Check sheet for the modelled part. Datum: model origin and axes. Units: mm. Round coordinates to 2 decimals unless told otherwise and drop trailing zeros. Order: outer loops, then holes, each group sorted by start corner. A loop starts at its lowest first (then second) coordinate and runs counter-clockwise, first axis right, second up.
(1) Sectioned sample at B-B, the plane y = 107. Enter the section's corners in (x, z), and give its area (3 significant figures).
(2) Thickness scan on probe 1 along X at (y, z) = (259, 5.75); probe 2 along Z at (x, y) = (-16.5, 148). Record the ranges inside material, lowest first.
(3) Sectioned sample at A-A, the plane z = 4.75. Enter the section's corners in (x, y).
(4) Depth check by flat-ended pin: pin 1 (2.5 mm diameter, centred on y = 215, z = 6.5, fed in from -X); pin 2 (1.9 mm diameter, centred on x = -11, y = 158.5, fed in from +Z). Enter the tip coordinate at first touch or a pass-through.
```python
from build123d import *

# Parameters (mm, degrees)
F1_DEPTH = 300
F2_W     = 5.8
F2_H     = 5.8
F3_DEPTH = 3.501


with BuildPart() as f1:
    # F0 (on Front) → F1 (new body)
    with BuildSketch(Plane.XZ):
        Polygon((-20.152273, 3.5), (-20.152273, 0), (19.247727, 0), (19.247727, 3.5), (15.247727, 3.5), (15.247727, 8.2), (13.247727, 8.2), (13.247727, 3.5), (7.047727, 3.5), (7.047727, 8.2), (-7.952273, 8.2), (-7.952273, 3.5), (-14.152273, 3.5), (-14.152273, 8.2), (-16.152273, 8.2), (-16.152273, 3.5), align=None)
    extrude(amount=-F1_DEPTH)

    # F2 (on face) → F3 (cut, through all)
    with BuildSketch(Plane.XY.offset(3.5)):
        with Locations((-11.252273, 26.756441)):
            Rectangle(F2_W, F2_H)
        with Locations((-11.252273, 73.556441)):
            Rectangle(F2_W, F2_H)
        with Locations((-11.252273, 120.356441)):
            Rectangle(F2_W, F2_H)
        with Locations((-11.252273, 167.156441)):
            Rectangle(F2_W, F2_H)
        with Locations((-11.252273, 213.956441)):
            Rectangle(F2_W, F2_H)
        with Locations((-11.252273, 260.756441)):
            Rectangle(F2_W, F2_H)
        with Locations((-11.252273, 307.556441)):
            Rectangle(F2_W, F2_H)
        with Locations((-11.252273, 354.356441)):
            Rectangle(F2_W, F2_H)
        with Locations((-11.252273, 401.156441)):
            Rectangle(F2_W, F2_H)
        with Locations((-11.252273, 447.956441)):
            Rectangle(F2_W, F2_H)
        with Locations((-11.252273, 494.756441)):
            Rectangle(F2_W, F2_H)
        with Locations((-11.252273, 541.556441)):
            Rectangle(F2_W, F2_H)
        with Locations((-11.252273, 588.356441)):
            Rectangle(F2_W, F2_H)
        with Locations((-11.252273, 635.156441)):
            Rectangle(F2_W, F2_H)
        with Locations((-11.252273, 681.956441)):
            Rectangle(F2_W, F2_H)
        with Locations((-11.252273, 728.756441)):
            Rectangle(F2_W, F2_H)
        with Locations((-11.252273, 775.556441)):
            Rectangle(F2_W, F2_H)
        with Locations((-11.252273, 822.356441)):
            Rectangle(F2_W, F2_H)
        with Locations((-11.252273, 869.156441)):
            Rectangle(F2_W, F2_H)
        with Locations((-11.252273, 915.956441)):
            Rectangle(F2_W, F2_H)
        with Locations((-11.252273, 962.756441)):
            Rectangle(F2_W, F2_H)
        with Locations((-11.252273, 1009.556441)):
            Rectangle(F2_W, F2_H)
        with Locations((-11.252273, 1056.356441)):
            Rectangle(F2_W, F2_H)
        with Locations((-11.252273, 1103.156441)):
            Rectangle(F2_W, F2_H)
        with Locations((-11.252273, 1149.956441)):
            Rectangle(F2_W, F2_H)
        with Locations((-11.252273, 1196.756441)):
            Rectangle(F2_W, F2_H)
        with Locations((-11.252273, 1243.556441)):
            Rectangle(F2_W, F2_H)
        with Locations((-11.252273, 1290.356441)):
            Rectangle(F2_W, F2_H)
        with Locations((-11.252273, 1337.156441)):
            Rectangle(F2_W, F2_H)
        with Locations((-11.252273, 1383.956441)):
            Rectangle(F2_W, F2_H)
        with Locations((10.347727, 26.756441)):
            Rectangle(F2_W, F2_H)
        with Locations((10.347727, 73.556441)):
            Rectangle(F2_W, F2_H)
        with Locations((10.347727, 120.356441)):
            Rectangle(F2_W, F2_H)
        with Locations((10.347727, 167.156441)):
            Rectangle(F2_W, F2_H)
        with Locations((10.347727, 213.956441)):
            Rectangle(F2_W, F2_H)
        with Locations((10.347727, 260.756441)):
            Rectangle(F2_W, F2_H)
        with Locations((10.347727, 307.556441)):
            Rectangle(F2_W, F2_H)
        with Locations((10.347727, 354.356441)):
            Rectangle(F2_W, F2_H)
        with Locations((10.347727, 401.156441)):
            Rectangle(F2_W, F2_H)
        with Locations((10.347727, 447.956441)):
            Rectangle(F2_W, F2_H)
        with Locations((10.347727, 494.756441)):
            Rectangle(F2_W, F2_H)
        with Locations((10.347727, 541.556441)):
            Rectangle(F2_W, F2_H)
        with Locations((10.347727, 588.356441)):
            Rectangle(F2_W, F2_H)
        with Locations((10.347727, 635.156441)):
            Rectangle(F2_W, F2_H)
        with Locations((10.347727, 681.956441)):
            Rectangle(F2_W, F2_H)
        with Locations((10.347727, 728.756441)):
            Rectangle(F2_W, F2_H)
        with Locations((10.347727, 775.556441)):
            Rectangle(F2_W, F2_H)
        with Locations((10.347727, 822.356441)):
            Rectangle(F2_W, F2_H)
        with Locations((10.347727, 869.156441)):
            Rectangle(F2_W, F2_H)
        with Locations((10.347727, 915.956441)):
            Rectangle(F2_W, F2_H)
        with Locations((10.347727, 962.756441)):
            Rectangle(F2_W, F2_H)
        with Locations((10.347727, 1009.556441)):
            Rectangle(F2_W, F2_H)
        with Locations((10.347727, 1056.356441)):
            Rectangle(F2_W, F2_H)
        with Locations((10.347727, 1103.156441)):
            Rectangle(F2_W, F2_H)
        with Locations((10.347727, 1149.956441)):
            Rectangle(F2_W, F2_H)
        with Locations((10.347727, 1196.756441)):
            Rectangle(F2_W, F2_H)
        with Locations((10.347727, 1243.556441)):
            Rectangle(F2_W, F2_H)
        with Locations((10.347727, 1290.356441)):
            Rectangle(F2_W, F2_H)
        with Locations((10.347727, 1337.156441)):
            Rectangle(F2_W, F2_H)
        with Locations((10.347727, 1383.956441)):
            Rectangle(F2_W, F2_H)
        with Locations((-11.252273, 1430.756441)):
            Rectangle(F2_W, F2_H)
        with Locations((-11.252273, 1477.556441)):
            Rectangle(F2_W, F2_H)
        with Locations((-11.252273, 1524.356441)):
            Rectangle(F2_W, F2_H)
        with Locations((-11.252273, 1571.156441)):
            Rectangle(F2_W, F2_H)
        with Locations((-11.252273, 1617.956441)):
            Rectangle(F2_W, F2_H)
        with Locations((-11.252273, 1664.756441)):
            Rectangle(F2_W, F2_H)
        with Locations((-11.252273, 1711.556441)):
            Rectangle(F2_W, F2_H)
        with Locations((-11.252273, 1758.356441)):
            Rectangle(F2_W, F2_H)
        with Locations((-11.252273, 1805.156441)):
            Rectangle(F2_W, F2_H)
        with Locations((-11.252273, 1851.956441)):
            Rectangle(F2_W, F2_H)
        with Locations((-11.252273, 1898.756441)):
            Rectangle(F2_W, F2_H)
        with Locations((-11.252273, 1945.556441)):
            Rectangle(F2_W, F2_H)
        with Locations((-11.252273, 1992.356441)):
            Rectangle(F2_W, F2_H)
        with Locations((-11.252273, 2039.156441)):
            Rectangle(F2_W, F2_H)
        with Locations((-11.252273, 2085.956441)):
            Rectangle(F2_W, F2_H)
        with Locations((-11.252273, 2132.756441)):
            Rectangle(F2_W, F2_H)
        with Locations((-11.252273, 2179.556441)):
            Rectangle(F2_W, F2_H)
        with Locations((-11.252273, 2226.356441)):
            Rectangle(F2_W, F2_H)
        with Locations((-11.252273, 2273.156441)):
            Rectangle(F2_W, F2_H)
        with Locations((-11.252273, 2319.956441)):
            Rectangle(F2_W, F2_H)
        with Locations((10.347727, 1430.756441)):
            Rectangle(F2_W, F2_H)
        with Locations((10.347727, 1477.556441)):
            Rectangle(F2_W, F2_H)
        with Locations((10.347727, 1524.356441)):
            Rectangle(F2_W, F2_H)
        with Locations((10.347727, 1571.156441)):
            Rectangle(F2_W, F2_H)
        with Locations((10.347727, 1617.956441)):
            Rectangle(F2_W, F2_H)
        with Locations((10.347727, 1664.756441)):
            Rectangle(F2_W, F2_H)
        with Locations((10.347727, 1711.556441)):
            Rectangle(F2_W, F2_H)
        with Locations((10.347727, 1758.356441)):
            Rectangle(F2_W, F2_H)
        with Locations((10.347727, 1805.156441)):
            Rectangle(F2_W, F2_H)
        with Locations((10.347727, 1851.956441)):
            Rectangle(F2_W, F2_H)
        with Locations((10.347727, 1898.756441)):
            Rectangle(F2_W, F2_H)
        with Locations((10.347727, 1945.556441)):
            Rectangle(F2_W, F2_H)
        with Locations((10.347727, 1992.356441)):
            Rectangle(F2_W, F2_H)
        with Locations((10.347727, 2039.156441)):
            Rectangle(F2_W, F2_H)
        with Locations((10.347727, 2085.956441)):
            Rectangle(F2_W, F2_H)
        with Locations((10.347727, 2132.756441)):
            Rectangle(F2_W, F2_H)
        with Locations((10.347727, 2179.556441)):
            Rectangle(F2_W, F2_H)
        with Locations((10.347727, 2226.356441)):
            Rectangle(F2_W, F2_H)
        with Locations((10.347727, 2273.156441)):
            Rectangle(F2_W, F2_H)
        with Locations((10.347727, 2319.956441)):
            Rectangle(F2_W, F2_H)
    extrude(amount=-F3_DEPTH, mode=Mode.SUBTRACT)


solid = f1.part
```
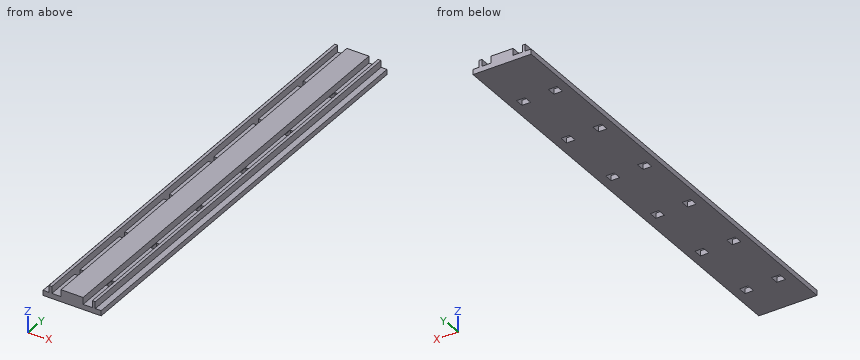
Derived:
1. outline: (-20.15, 0) - (19.25, 0) - (19.25, 3.5) - (15.25, 3.5) - (15.25, 8.2) - (13.25, 8.2) - (13.25, 3.5) - (7.05, 3.5) - (7.05, 8.2) - (-7.95, 8.2) - (-7.95, 3.5) - (-14.15, 3.5) - (-14.15, 8.2) - (-16.15, 8.2) - (-16.15, 3.5) - (-20.15, 3.5) - close
1. area: 227 mm2
2. probe 1: x = -16.15 to -14.15, -7.95 to 7.05, 13.25 to 15.25
2. probe 2: z = 0 to 3.5
3. outline: (-16.15, 0) - (-14.15, 0) - (-14.15, 300) - (-16.15, 300) - close; (-7.95, 0) - (7.05, 0) - (7.05, 300) - (-7.95, 300) - close; (13.25, 0) - (15.25, 0) - (15.25, 300) - (13.25, 300) - close
4. pin 1: stops at x = -16.15
4. pin 2: stops at z = 3.5
